Solid Edge part; units mm, degrees
sketch "Sketch1" plane through (0, 0, 0) normal (0, -1, 0) x (1, 0, 0)
  circle A0 centre (0, 0) radius 1.5875
extrude "Protrusion1" add sketch "Sketch1" along normal blind 19.05
sketch "Sketch2" plane through (0, -19.05, 0) normal (0, -1, 0) x (1, 0, 0)
  circle A0 centre (0, 0) radius 3.1115
extrude "ExtrudedProtrusion_2" add sketch "Sketch2" along normal blind 2.2606
fillet "Round_1" radius 1.27 1 edges at (-3.1115, -21.3106, 0)
cosmetic_thread "Thread1"
properties part number "90272A130"
Read the model definition and answer for the solid it produces. Units are mm, in the model's axes. A direction names the side the tool comes from. Give positions to 0.01 mm unless a question says otherwise; leave off trailing zeros. Order: outer loops, then holes, each group sorted by start corner. A loop starts at its lowest first (then second) coordinate and runs counter-clockwise, first axis right, second up.
(1) Find section A-A (x = 0). Give the vertices of the cut face in (y, z), plus the area to 3 significant figures.
(2) Find section C-C (y = -7.75). Give the vertices of the cut face in (x, z) (1 decimal).
(3) Find section B-B (z = 0). Give the vertices of the cut face in (x, y), plus the area to 3 significant figures.
(4) Given pin 1 (2 mm diameter, centred on x = 0, y = -13, fed in from +Z); pin 2 (2 mm diameter, centred on y = -18.5, z = -1.5, fed in from +X); pin 3 (2 mm diameter, centred on y = -11.5, z = -1, fed in from -X), each flat-ended and moving along its own axis, determine where each tip first touches the part or whether it passes through.
(5) For faces 1 (the flat face through (0, 0, 0)), 2 (the flat face through (-1.3, -19.05, -1.3)), determine the directions among +Z, -Z, +X, -X, +Y, -Y from which every point of the face is accessible in a straight line to the end or side of a thin tool.
(6) Straight lines are drawn through the part: L1, parallel to X at y = -19.5, z = 2.25; L2, parallel to Z at x = -0.25, y = -3.25; L3, parallel to Z at x = 1.25, y = -17. For each, find the intervals that lie inside material, in ascending order.
Result sheet:
1. outline: (-21.31, -1.84) arc R1.27 ccw to (-20.04, -3.11) - (-19.05, -3.11) - (-19.05, -1.59) - (0, -1.59) - (0, 1.59) - (-19.05, 1.59) - (-19.05, 3.11) - (-20.04, 3.11) arc R1.27 ccw to (-21.31, 1.84) - close
1. area: 73.9 mm2
2. outline: circle Ø3.2 at (0, 0)
3. outline: (-3.11, -20.04) arc R1.27 ccw to (-1.84, -21.31) - (1.84, -21.31) arc R1.27 ccw to (3.11, -20.04) - (3.11, -19.05) - (1.59, -19.05) - (1.59, 0) - (-1.59, 0) - (-1.59, -19.05) - (-3.11, -19.05) - close
3. area: 73.9 mm2
4. pin 1: stops at z = 1.59
4. pin 2: stops at x = 3.04
4. pin 3: stops at x = -1.59
5. face 1: +Z, -Z, +X, -X, +Y
5. face 2: +Y
6. L1: x = -2.15 to 2.15
6. L2: z = -1.57 to 1.57
6. L3: z = -0.98 to 0.98
